Autodesk Inventor part; units mm, degrees
ref_plane "YZ Plane" through (0, 0, 0) normal (1, 0, 0) x (0, 1, 0)
ref_plane "XZ Plane" through (0, 0, 0) normal (0, 1, 0) x (-1, 0, 0)
ref_plane "XY Plane" through (0, 0, 0) normal (0, 0, 1) x (1, 0, 0)
sketch "Sketch1" plane through (0, 0, 0) normal (1, 0, 0) x (0, 1, 0)
  line L0 (0, 0) -> (171.45, 0)
  line L1 (171.45, 0) -> (171.45, -271.78)
  line L2 (171.45, -271.78) -> (0, -271.78)
  line L3 (0, -271.78) -> (0, 0)
  line L4 (0, 0) -> (53.34, 0)
  line L5 (53.34, 0) -> (53.34, -271.78)
  line L6 (53.34, 0) -> (171.45, -42.9885)
  line L7 (53.34, 0) -> (179.03, 0) construction
  line L8 (173.99, -274.32) -> (173.99, 2.54)
  line L9 (173.99, 2.54) -> (-2.54, 2.54)
  line L10 (-2.54, 2.54) -> (-2.54, -274.32)
  line L11 (-2.54, -274.32) -> (173.99, -274.32)
  line L12 (54.2087, 2.3868) -> (172.3187, -40.6017)
  line L13 (179.03, -43.0444) -> (43.4558, 6.3006)
  point P0 (53.7879, 2.54)
  point P1 (173.99, -41.21)
  dimension "d0" = 171.45
  dimension "d1" = 271.78
  dimension "d2" = 53.34
  dimension "d3" = 20
  dimension "d4" = 2.54
  dimension "d5" = 2.54
extrude "Extrusion1" add sketch "Sketch1" along normal blind 121.92 contours L3 L2 L1 L12 L13 L8 L11 L10 L9 L0 | L0 L12 L1 L6
sketch "Sketch2" plane through (121.92, 0, 0) normal (1, 0, 0) x (0, 0, -1)
  line L0 (0, 0) -> (0, 53.34)
  line L1 (0, 53.34) -> (271.78, 53.34)
  line L2 (271.78, 171.45) -> (271.78, 0)
  line L3 (271.78, 55.88) -> (-2.54, 55.88)
  line L4 (-2.54, 55.88) -> (-2.54, 0)
  line L5 (0, 53.34) -> (42.9885, 171.45)
  line L6 (5.0738, 67.2802) -> (-1.6206, 48.8875)
  line L7 (271.78, 82.1996) -> (271.78, 27.94)
  point P0 (0.9245, 55.88)
  dimension "d8" = 2.54
extrude "Extrusion2" add sketch "Sketch2" against normal blind 121.92
sketch "Sketch3" plane through (0, -2.54, -274.32) normal (0, 0, -1) x (-1, 0, 0)
  line L0 (0, 0) -> (-121.92, 0)
  line L1 (-121.92, 0) -> (0, 0)
  line L2 (-121.92, 55.88) -> (0, 55.88)
  line L3 (0, 0) -> (0, 55.88)
  line L4 (0, 55.88) -> (-121.92, 55.88)
  line L5 (0, 58.42) -> (-121.92, 58.42)
  line L6 (-121.92, 55.88) -> (-121.92, 0)
  circle A0 centre (-60.96, 27.94) radius 27.94
  line L7 (-83.46, 13.94) -> (-38.46, 13.94)
  line L8 (-38.46, 13.94) -> (-38.46, 41.94)
  line L9 (-38.46, 41.94) -> (-83.46, 41.94)
  line L10 (-83.46, 41.94) -> (-83.46, 13.94)
  line L11 (-83.46, 13.94) -> (-38.46, 41.94) construction
  line L12 (-38.46, 13.94) -> (-83.46, 41.94) construction
  line L13 (-60.9761, 7.94) -> (-60.9439, 7.94)
  line L14 (-60.9439, 47.94) -> (-60.9761, 47.94)
  line L15 (-60.9761, 7.94) -> (-60.9439, 47.94) construction
  line L16 (-60.9439, 7.94) -> (-60.9761, 47.94) construction
  circle A1 centre (-60.96, 47.94) radius 1.8
  circle A2 centre (-60.96, 7.94) radius 1.8
  line L17 (-60.9761, 47.94) -> (-60.9761, 46.1401)
  line L18 (-60.9439, 46.1401) -> (-60.9439, 47.94)
  line L19 (-60.9761, 41.94) -> (-60.9761, 13.94)
  line L20 (-60.9761, 9.7399) -> (-60.9761, 7.94)
  line L21 (-60.9439, 7.94) -> (-60.9439, 9.7399)
  line L22 (-60.9439, 13.94) -> (-60.9439, 41.94)
  point P0 (0, 2.54)
  dimension "d11" = 45
  dimension "d12" = 28
  dimension "d13" = 40
  dimension "d14" = 3.6
extrude "Extrusion3" cut sketch "Sketch3" against normal blind 121.92 contours L10 L9 L19 L7 | L19 L9 L22 L7 | L22 L9 L8 L7 | L20 A2 L21 L13 | L13 L21 A2 L20 | L18 A1 L17 L14 | L14 L17 A1 L18
sketch "Sketch4" plane through (0, -2.54, -274.32) normal (0, 0, -1) x (-1, 0, 0)
  line L0 (-38.46, 41.94) -> (-38.46, 13.94)
  line L1 (-83.46, 13.94) -> (-83.46, 41.94)
  line L2 (-38.46, 41.94) -> (-83.46, 41.94)
  line L3 (-83.46, 41.94) -> (-83.46, 13.94)
  line L4 (-83.46, 13.94) -> (-38.46, 13.94)
  line L5 (-38.46, 13.94) -> (-38.46, 41.94)
  line L6 (-86.36, 13.94) -> (-35.56, 13.94)
  line L7 (-35.56, 13.94) -> (-35.56, 41.94)
  line L8 (-35.56, 41.94) -> (-86.36, 41.94)
  line L9 (-86.36, 41.94) -> (-86.36, 13.94)
  line L10 (-86.36, 13.94) -> (-35.56, 41.94) construction
  line L11 (-35.56, 13.94) -> (-86.36, 41.94) construction
  point P0 (0, 2.54)
  point P1 (-60.96, 27.94)
  dimension "d17" = 50.8
extrude "Extrusion4" cut sketch "Sketch4" against normal blind 121.92 contours L8 L7 L6 L0 | L1 L6 L9 L8
sketch "Sketch5" plane through (121.92, 0, 0) normal (1, 0, 0) x (0, 0, -1)
  line L0 (271.78, 53.34) -> (271.78, 0)
  line L1 (271.78, 53.34) -> (246.38, 53.34)
  line L2 (271.78, 53.34) -> (0, 53.34)
  line L3 (246.38, 53.34) -> (246.38, 43.18)
  line L4 (246.38, 43.18) -> (272.1958, 43.18)
  line L5 (246.38, 43.18) -> (226.8063, 53.34)
  line L6 (226.8063, 53.34) -> (209.4202, 62.3644)
  line L7 (245.2098, 40.9256) -> (225.6361, 51.0856)
  line L8 (225.6361, 51.0856) -> (208.25, 60.1101)
  line L9 (246.38, 40.64) -> (272.1958, 40.64)
  line L10 (239.3965, 43.9431) -> (259.2879, 33.6182)
  line L11 (267.1647, 40.64) -> (232.6379, 40.64)
  point P0 (0, 0)
  point P1 (245.7601, 40.64)
  point P2 (271.78, 40.64)
  point P3 (271.78, 43.18)
  point P4 (221.2929, 53.34)
  dimension "d20" = 25.4
  dimension "d21" = 10.16
  dimension "d22" = 2.54
  dimension "d23" = 2.54
extrude "Extrusion5" add sketch "Sketch5" against normal blind 121.92 contours L0 L9 L11 L10 L7 L8 L2 L5 L4
sketch "Sketch6" plane through (0, 0, 0) normal (-1, 0, 0) x (0, 0, 1)
  line L0 (-226.8063, 53.34) -> (-246.38, 43.18)
  line L1 (-233.7398, 49.741) -> (-197.786, 68.4033)
  line L2 (-197.786, 68.4033) -> (-271.78, 69.3117)
  line L3 (-271.78, 171.45) -> (-271.78, 55.88)
  line L4 (-271.78, 69.3117) -> (-271.78, 47.3341)
  line L5 (-271.78, 53.34) -> (-271.78, 43.18)
  line L6 (-271.78, 47.3341) -> (-233.7398, 49.741)
  point P0 (0, 0)
extrude "Extrusion6" cut sketch "Sketch6" against normal blind 121.92
sketch "Sketch7" plane through (121.92, 0, 0) normal (1, 0, 0) x (0, 0, -1)
  line L0 (-2.54, -2.54) -> (274.32, -2.54)
  line L1 (274.32, 173.99) -> (41.21, 173.99)
  line L2 (-2.54, -2.54) -> (274.32, -2.54)
  line L3 (274.32, -2.54) -> (274.32, 173.99)
  line L4 (274.32, 173.99) -> (-2.54, 173.99)
  line L5 (-2.54, 173.99) -> (-2.54, -2.54)
  line L6 (41.21, 173.99) -> (-2.54, 53.7879)
  line L7 (41.21, 173.99) -> (-2.54, 53.7879)
  point P0 (0, 0)
extrude "Extrusion7" add sketch "Sketch7" along normal blind 2.54 contours L5 L6 L1 L3 L0
sketch "Sketch8" plane through (0, -2.54, -274.32) normal (0, 0, -1) x (-1, 0, 0)
  line L0 (0, 173.99) -> (-121.92, 173.99)
  line L1 (-121.92, 173.99) -> (0, 173.99)
  line L2 (0, 173.99) -> (0, 52.07)
  line L3 (0, 52.07) -> (-121.92, 52.07)
  line L4 (-121.92, 52.07) -> (-121.92, 173.99)
  circle A0 centre (-60.96, 113.03) radius 57.15
  point P0 (0, 2.54)
  dimension "d30" = 121.92
  dimension "d31" = 114.3
extrude "Extrusion8" cut sketch "Sketch8" against normal blind 25.4 contours A0
properties part number "Electronics Case for Bubba"
Part model, mm, in its own coordinate system. A direction names the side the tool comes from. Coordinates: 2 decimals unless noted, no trailing zeros. Write each loop counter-clockwise with the first axis right and the second up, starting at its lowest first coordinate (ties: lowest second). Pieces come first, ordered by that corner, then holes.
Item 1: Pin check, flat tips, straight feed: pin 1 (3 mm diameter, centred on x = 60.96, y = 45.4, fed in from -Z); pin 2 (0.8 mm diameter, centred on y = 18.5, z = -273.5, fed in from -X); pin 3 (10 mm diameter, centred on x = 32, y = 112, fed in from -Z); pin 4 (12 mm diameter, centred on y = 82, z = -115, fed in from -X). Stop position of each tip, or through.
Item 2: Slice it at B-B (z = -90.5). Write the cut outline in (x, y).
Item 3: Slice it at C-C (x = 115). Write the cut outline in (y, z), and give its area (3 significant figures).
Item 4: Probe line 1 (Y direction, x = 36, z = -82.5); line 2 (Z direction, x = 96, y = 19); line 3 (Y direction, x = 8.5, z = -240.5). List the from-to ranges inside material, lowest first.
Item 5: Slice it at A-A (y = 110.49). Write the cut outline in (x, z).
Item 6: Which spindle directions (+Z, -Z, +X, -X, +Y, -Y) get a long thin tool onto all of the face, cutting with end or side? Do faces 1 (the face through (61, -2.54, -134)), 2 (the face through (8.17, 88.6, -273.07)), 3 (the face through (62, 53.34, -109)). Say none if no direction does.
Item 7: Mould opens along Z. For faces 4 (the face through (124.46, 87, -134)), 5 (the face through (62, 55.88, -113)), 6 (the face through (75, 45, -274.32)) say: released by +Z, released by -Z, zero draft, split by the parting line, or undercut.
Results found:
1. pin 1: stops at z = -244.99
1. pin 2: stops at x = 0
1. pin 3: stops at z = -23.17
1. pin 4: stops at x = 121.92
2. outline: (0, -2.54) - (124.46, -2.54) - (124.46, 173.99) - (0, 173.99) - (0, 171.45) - (121.92, 171.45) - (121.92, 55.88) - (0, 55.88) - (0, 53.34) - (121.92, 53.34) - (121.92, 0) - (0, 0) - close
3. outline: (-2.54, -274.32) - (91.89, -274.32) - (91.89, -271.78) - (43.18, -271.78) - (43.18, -246.38) - (53.34, -226.81) - (55.88, -221.91) - (55.88, -0.92) - (171.45, -42.99) - (171.45, -271.78) - (129.09, -271.78) - (129.09, -274.32) - (173.99, -274.32) - (173.99, -41.21) - (172.32, -40.6) - (54.21, 2.39) - (53.79, 2.54) - (-2.54, 2.54) - close; hole (0, -271.78) - (40.64, -271.78) - (40.64, -245.76) - (40.93, -245.21) - (51.09, -225.64) - (53.34, -221.29) - (53.34, 0) - (0, 0) - close
3. area: 2,790 mm2
4. line 1: y = -2.54 to 0, 53.34 to 55.88, 171.45 to 173.99
4. line 2: z = -274.32 to -271.78, 0 to 2.54
4. line 3: y = -2.54 to 0, 43.37 to 46.23, 171.45 to 173.99
5. outline: (0, -274.32) - (3.81, -274.32) - (3.81, -271.78) - (0, -271.78) - close; (0, -20.8) - (121.92, -20.8) - (121.92, -271.78) - (118.11, -271.78) - (118.11, -274.32) - (124.46, -274.32) - (124.46, -18.1) - (0, -18.1) - close
6. face 1: +Z, -Z, +X, -X, -Y
6. face 2: -Z
6. face 3: -X
7. face 4: zero draft
7. face 5: undercut
7. face 6: released by -Z
